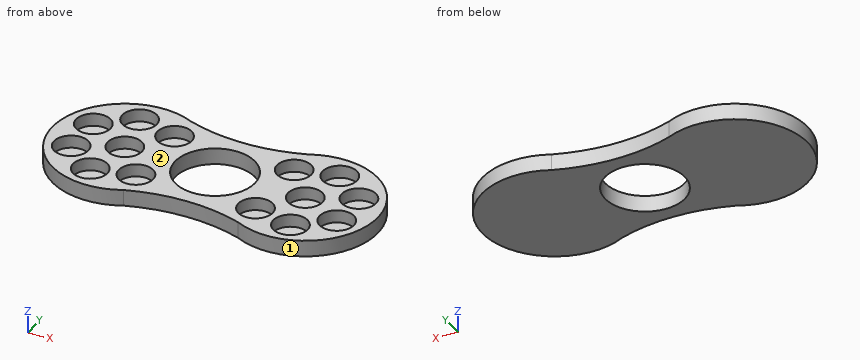
```python
from build123d import *

# Parameters (mm, degrees)
F0_R     = 4.75
F0_R_2   = 11
F1_DEPTH = 4.5
F2_DEPTH = 1


# Not quite as in the source:
# - a feature names something its author has since deleted; it is built from what else it names


with BuildPart() as f1:
    # F0 (on Top) → F1 (new body)
    with BuildSketch(Plane.XY):
        with BuildLine():
            ThreePointArc((-15.8212677669, -17.7693802535), (0, -15.0870091218), (15.8212677669, -17.7693802535))
            ThreePointArc((15.8212677669, -17.7693802535), (44.9980398453, -0.2800041916), (16.3223672692, 18.019397609))
            ThreePointArc((16.3223672692, 18.019397609), (0, 15.1589625906), (-16.3223672692, 18.019397609))
            ThreePointArc((-16.3223672692, 18.019397609), (-44.9980398453, -0.2800041916), (-15.8212677669, -17.7693802535))
        make_face()
        with Locations((-27.7271234226, -12.8301069662)):
            Circle(F0_R, mode=Mode.SUBTRACT)
        with Locations((-16.5687225704, -10.0480051668)):
            Circle(F0_R, mode=Mode.SUBTRACT)
        with Locations((-36.7892470891, -5.75)):
            Circle(F0_R, mode=Mode.SUBTRACT)
        with Locations((16.5687225704, -10.0480051668)):
            Circle(F0_R, mode=Mode.SUBTRACT)
        with Locations((27.7271234226, -12.8301069662)):
            Circle(F0_R, mode=Mode.SUBTRACT)
        with Locations((36.7892470891, -5.75)):
            Circle(F0_R, mode=Mode.SUBTRACT)
        with Locations((-25, 0)):
            Circle(F0_R, mode=Mode.SUBTRACT)
        with Locations((-36.7892470891, 5.75)):
            Circle(F0_R, mode=Mode.SUBTRACT)
        with Locations((-27.7271234226, 12.8301069662)):
            Circle(F0_R, mode=Mode.SUBTRACT)
        with Locations((-16.5687225704, 10.0480051668)):
            Circle(F0_R, mode=Mode.SUBTRACT)
        Circle(F0_R_2, mode=Mode.SUBTRACT)
        with Locations((25, 0)):
            Circle(F0_R, mode=Mode.SUBTRACT)
        with Locations((36.7892470891, 5.75)):
            Circle(F0_R, mode=Mode.SUBTRACT)
        with Locations((16.5687225704, 10.0480051668)):
            Circle(F0_R, mode=Mode.SUBTRACT)
        with Locations((27.7271234226, 12.8301069662)):
            Circle(F0_R, mode=Mode.SUBTRACT)
    extrude(amount=F1_DEPTH)

    # F0 (on Top) → F2 (join)
    with BuildSketch(Plane.XY):
        with Locations((-25, 0)):
            Circle(F0_R)
        with Locations((25, 0)):
            Circle(F0_R)
        with Locations((-16.5687225704, 10.0480051668)):
            Circle(F0_R)
        with Locations((-27.7271234226, 12.8301069662)):
            Circle(F0_R)
        with Locations((-36.7892470891, 5.75)):
            Circle(F0_R)
        with Locations((-36.7892470891, -5.75)):
            Circle(F0_R)
        with Locations((-27.7271234226, -12.8301069662)):
            Circle(F0_R)
        with Locations((-16.5687225704, -10.0480051668)):
            Circle(F0_R)
        with Locations((16.5687225704, 10.0480051668)):
            Circle(F0_R)
        with Locations((27.7271234226, 12.8301069662)):
            Circle(F0_R)
        with Locations((36.7892470891, 5.75)):
            Circle(F0_R)
        with Locations((36.7892470891, -5.75)):
            Circle(F0_R)
        with Locations((27.7271234226, -12.8301069662)):
            Circle(F0_R)
        with Locations((16.5687225704, -10.0480051668)):
            Circle(F0_R)
    extrude(amount=F2_DEPTH)


solid = f1.part
```
CAD build for the part. Positions are in the model's coordinates, mm. Face numbers are marked on the shaded views. Give positions to 0.01 mm unless a question says otherwise; leave off trailing zeros. Order: outer loops, then holes, each group sorted by start corner. A loop starts at its lowest first (then second) coordinate and runs counter-clockwise, first axis right, second up. Notation, with made-up numbers: M 69,11.5 L 120,11.5 A17 cw 120,26.5 Z; hole C 68,-20.5 d6. An arc over 180 degrees is marked long. Put each result on its own line as item: value. Start each with the question number.
(1) Saw through at A-A, the plane x = 0. Write the cut outline in (y, z).
(2) Saw through at B-B, the plane y = 0. Write the cut outline in (x, z), then the cut area to 4 significant figures.
(3) Flat gauge pins, fed straight in: pin 1 Ø7.5 at (x, y) = (-28, -13) entering from +Z; pin 2 Ø1 at (x, z) = (-15, 2.5) entering from -Y. Where does each tip first touch, or does it go through?
(4) Mould opens along X. For the marked faces 1 and 2 say: +X half, -X half, draft (parallel to the pull), parting line (faces both ways), or undercut.
(5) Saw through at C-C, the plane z = 2.2. Give the number of separate pieces and of enclosed holes in the cut face, then the cut area to 3 significant figures.
(6) Drill centre lines: line 1 along X through (y, z) = (11.5, 1.25); line 2 along Y through (x, z) = (23.5, 1.4); line 3 along Y through (x, z) = (20, 4.05). Where is each one in solid material? Low to high.
(7) Saw through at D-D, the plane x = -25. Write the cut outline in (y, z), then the cut area to 3 significant figures.
Check result:
1. outline: M -15.09,0 L -11,0 L -11,4.5 L -15.09,4.5 Z; M 11,0 L 15.16,0 L 15.16,4.5 L 11,4.5 Z
2. outline: M -45,0 L -11,0 L -11,4.5 L -20.25,4.5 L -20.25,1 L -29.75,1 L -29.75,4.5 L -45,4.5 Z; M 11,0 L 45,0 L 45,4.5 L 29.75,4.5 L 29.75,1 L 20.25,1 L 20.25,4.5 L 11,4.5 Z
2. area: 239.5 mm2
3. pin 1: stops at z = 1
3. pin 2: stops at y = -17.66
4. face 1: undercut
4. face 2: draft
5. separate pieces: 1
5. enclosed holes: 15
5. area: 1,600 mm2
6. line 1: x = -41.36 to -32.29, -23.17 to -21.09, -12.05 to 12.05, 21.09 to 23.17, 32.29 to 41.36
6. line 2: y = -19.94 to -15, -10.66 to -4.51, 4.51 to 10.66, 15 to 19.94
6. line 3: y = -19.36 to -13.33, -6.76 to 6.76, 13.33 to 19.36
7. outline: M -20,0 L 20,0 L 20,4.5 L 16.72,4.5 L 16.72,1 L 8.94,1 L 8.94,4.5 L 4.75,4.5 L 4.75,1 L -4.75,1 L -4.75,4.5 L -8.94,4.5 L -8.94,1 L -16.72,1 L -16.72,4.5 L -20,4.5 Z
7. area: 92.3 mm2
